Read the model definition and answer for the solid it produces. Units are mm, in the model's axes. A direction names the side the tool comes from. Coordinates: 2 decimals unless noted, no trailing zeros. Write each loop counter-clockwise with the first axis right and the second up, starting at its lowest first coordinate (ties: lowest second). Pieces come first, ordered by that corner, then holes. Notation, with made-up numbers: (34.25, 20) -> (52.25, 20) arc R10 ccw to (52.25, 36) -> close; hole circle Ø4 at (-38, 15). An arc over 180 degrees is marked (long way). Return JSON: item names as keys, results as strings.
from build123d import *

# Parameters (mm, degrees)
F2_DEPTH = 12.7


with BuildPart() as f2:
    # F0 (on Top) → F2 (new body, through all)
    with BuildSketch(Plane.XY):
        with BuildLine():
            Line((-20.507467, 31.75), (-17.952428, 44.894538))
            Line((-17.952428, 44.894538), (7.68059, 70.978887))
            ThreePointArc((7.68059, 70.978887), (7.617897, 78.162819), (0.433966, 78.100125))
            Line((0.433966, 78.100125), (-27.342302, 49.83479))
            Line((-27.342302, 49.83479), (-32.832533, 21.59))
            Line((-32.832533, 21.59), (-5.08, 21.59))
            Line((-5.08, 21.59), (-5.08, 0))
            ThreePointArc((-5.08, 0), (0, -5.08), (5.08, 0))
            Line((5.08, 0), (5.08, 31.75))
            Line((5.08, 31.75), (-20.507467, 31.75))
        make_face()
    extrude(amount=F2_DEPTH)


solid = f2.part
1. The part is cut by section B-B (z = 10). Determine the outline of the cut face in (x, y), then the cut area to 3 significant figures.
Taken from the geometry:
{"outline": "(-32.83, 21.59) -> (-5.08, 21.59) -> (-5.08, 0) arc R5.08 ccw to (5.08, 0) -> (5.08, 31.75) -> (-20.51, 31.75) -> (-17.95, 44.89) -> (7.68, 70.98) arc R5.08 ccw to (0.43, 78.1) -> (-27.34, 49.83) -> close", "area": "1,220 mm2"}
2. The part is cut by section D-D (x = -23). Determine the outline of the cut face in (y, z).
Taken from the geometry:
{"outline": "(21.59, 0) -> (54.25, 0) -> (54.25, 12.7) -> (21.59, 12.7) -> close"}
3. Consider L1, parallel to X at y = 5, z = 8.75; L2, parallel to Y at x = -17.5, z = 1; L3, parallel to Y at x = -14, z = 8.5. Determine where each line is inside the solid, lowest interval first.
Taken from the geometry:
{"L1": "x = -5.08 to 5.08", "L2": "y = 21.59 to 31.75, 45.35 to 59.85", "L3": "y = 21.59 to 31.75, 48.92 to 63.41"}
4. Flat-ended cylindrical pins translate along their axes: pin 1 Ø6 at (y, z) = (10, 2) entering from +X; pin 2 Ø5 at (y, z) = (62.5, 7) entering from -X; pin 3 Ø5 at (x, z) = (-11, 6.5) entering from +Y. Find the tip coordinate at first contact, or state that the pin passes through.
Taken from the geometry:
{"pin 1": "stops at x = 5.08", "pin 2": "stops at x = -17.35", "pin 3": "stops at y = 69.01"}
5. The part is cut by section C-C (y = 15). Determine the outline of the cut face in (x, z).
Taken from the geometry:
{"outline": "(-5.08, 0) -> (5.08, 0) -> (5.08, 12.7) -> (-5.08, 12.7) -> close"}
6. The part is cut by section A-A (x = -17). Determine the outline of the cut face in (y, z).
Taken from the geometry:
{"outline": "(21.59, 0) -> (31.75, 0) -> (31.75, 12.7) -> (21.59, 12.7) -> close; (45.86, 0) -> (60.36, 0) -> (60.36, 12.7) -> (45.86, 12.7) -> close"}
7. A tool of negligible diameter and unlimited length cuts with its end or side. For faces 1 (the face through (-13.26, 64.165, 6.261)), 2 (the face through (-19, 21.59, 6)), 3 (the face through (-19.248, 38.23, 6.261)), 4 (the face through (5.08, 16, 6)), from which of +Z, -Z, +X, -X, +Y, -Y can it reach the whole face along a straight path? Write none if from no direction.
Taken from the geometry:
{"face 1": "+Z, -Z, -X, +Y", "face 2": "+Z, -Z, -X, -Y", "face 3": "+Z, -Z, +X", "face 4": "+Z, -Z, +X, -Y"}
